The model under review builds one solid part; all positions refer to its coordinate system, in mm. A direction names the side the tool comes from. Round coordinates to 2 decimals unless told otherwise and drop trailing zeros. Write each loop counter-clockwise with the first axis right and the second up, starting at its lowest first coordinate (ties: lowest second). Pieces come first, ordered by that corner, then holes. Notation, with made-up numbers: (34, 41.25) - (63, 41.25) arc R16 ccw to (63, 70.25) - close; hole circle Ø2 at (3.5, -16). An arc over 180 degrees is marked (long way). Use one line per item in the form item = value.
from build123d import *

# Parameters (mm, degrees)
SKETCH_1_R                = 27.5
EXTRUDE_1_DEPTH           = 60
EXTRUDE_1_DEPTH_BACK      = 50
SKETCH_10_W               = 6
SKETCH_10_H               = 40
CUT_EXTRUDE_8_DEPTH       = 8.1
SKETCH_10_2_W             = 6
SKETCH_10_2_H             = 40
CUT_EXTRUDE_9_DEPTH       = 10
CUT_EXTRUDE_9_DEPTH_BACK  = 10
CUT_EXTRUDE_10_DEPTH      = 54
SKETCH_12_R               = 26.5
CUT_EXTRUDE_11_DEPTH      = 58
CUT_EXTRUDE_11_DEPTH_BACK = 54
SKETCH_13_W               = 13
SKETCH_13_H               = 23.5
CUT_EXTRUDE_12_DEPTH      = 54
SKETCH_14_W               = 5
SKETCH_14_H               = 5
EXTRUDE_2_DEPTH           = 1
EXTRUDE_2_DEPTH_BACK      = 4
SKETCH_15_R               = 1.15
CUT_EXTRUDE_13_DEPTH      = 4
CUT_EXTRUDE_13_DEPTH_BACK = 5


with BuildPart() as part:
    # Sketch 1 → Extrude 1 (new body, two sides)
    with BuildSketch(Plane(origin=(0, 0, 0), x_dir=(1, 0, 0), z_dir=(0, 1, 0))) as extrude_1_sk:
        Circle(SKETCH_1_R)
    extrude(amount=EXTRUDE_1_DEPTH)
    extrude(extrude_1_sk.sketch, amount=-EXTRUDE_1_DEPTH_BACK)

    # Sketch 10 → Cut-Extrude 8 (cut)
    with BuildSketch(Plane(origin=(0, 60, 0), x_dir=(1, 0, 0), z_dir=(0, 1, 0))):
        with Locations((-12, 0)):
            Rectangle(SKETCH_10_W, SKETCH_10_H)
        with Locations((12, 0)):
            Rectangle(SKETCH_10_W, SKETCH_10_H)
    extrude(amount=-CUT_EXTRUDE_8_DEPTH, mode=Mode.SUBTRACT)

    # Sketch 10_2 → Cut-Extrude 9 (cut, two sides)
    with BuildSketch(Plane(origin=(0, 60, 0), x_dir=(1, 0, 0), z_dir=(0, 1, 0))) as cut_extrude_9_sk:
        with Locations((-12, 0)):
            Rectangle(SKETCH_10_2_W, SKETCH_10_2_H)
        with Locations((12, 0)):
            Rectangle(SKETCH_10_2_W, SKETCH_10_2_H)
    extrude(amount=CUT_EXTRUDE_9_DEPTH, mode=Mode.SUBTRACT)
    extrude(cut_extrude_9_sk.sketch, amount=-CUT_EXTRUDE_9_DEPTH_BACK, mode=Mode.SUBTRACT)

    # Sketch 11 → Cut-Extrude 10 (cut)
    with BuildSketch(Plane(origin=(0, 0, 0), x_dir=(1, 0, 0), z_dir=(0, 1, 0))):
        with BuildLine():
            Line((23.587956714, 14.137124816), (-24.13203639, 13.186918505))
            ThreePointArc((-24.13203639, 13.186918505), (0.547474823, -27.494549848), (23.587956714, 14.137124816))
        make_face()
    extrude(amount=-CUT_EXTRUDE_10_DEPTH, mode=Mode.SUBTRACT)

    # Sketch 12 → Cut-Extrude 11 (cut, two sides)
    with BuildSketch(Plane(origin=(0, 0, 0), x_dir=(1, 0, 0), z_dir=(0, 1, 0))) as cut_extrude_11_sk:
        Circle(SKETCH_12_R)
    extrude(amount=CUT_EXTRUDE_11_DEPTH, mode=Mode.SUBTRACT)
    extrude(cut_extrude_11_sk.sketch, amount=-CUT_EXTRUDE_11_DEPTH_BACK, mode=Mode.SUBTRACT)

    # Sketch 13 → Cut-Extrude 12 (cut)
    with BuildSketch(Plane.XY):
        with Locations((0, -24.25)):
            Rectangle(SKETCH_13_W, SKETCH_13_H)
    extrude(amount=-CUT_EXTRUDE_12_DEPTH, mode=Mode.SUBTRACT)

    # Sketch 14 → Extrude 2 (add, two sides)
    with BuildSketch(Plane.XY.offset(-28)) as extrude_2_sk:
        with Locations((0, -38.5)):
            Rectangle(SKETCH_14_W, SKETCH_14_H)
        with Locations((0, -10)):
            Rectangle(SKETCH_14_W, SKETCH_14_H)
    extrude(amount=EXTRUDE_2_DEPTH)
    extrude(extrude_2_sk.sketch, amount=-EXTRUDE_2_DEPTH_BACK)

    # Sketch 15 → Cut-Extrude 13 (cut, two sides)
    with BuildSketch(Plane.XY.offset(-28)) as cut_extrude_13_sk:
        with Locations((0, -10)):
            Circle(SKETCH_15_R)
        with Locations((0, -38.5)):
            Circle(SKETCH_15_R)
    extrude(amount=CUT_EXTRUDE_13_DEPTH, mode=Mode.SUBTRACT)
    extrude(cut_extrude_13_sk.sketch, amount=-CUT_EXTRUDE_13_DEPTH_BACK, mode=Mode.SUBTRACT)


solid = part.part
(1) Add section B-B on y = -33.5. Write out the cut boundary in (x, z).
Geometry results:
outline = (-24.13, -13.19) arc R27.5 ccw to (-6.5, -26.72) - (-6.5, -25.69) arc R26.5 cw to (-22.97, -13.21) - close; (6.5, -26.72) arc R27.5 ccw to (23.59, -14.14) - (22.43, -14.11) arc R26.5 cw to (6.5, -25.69) - close
(2) Add section A-A on z = 0. Write out the cut boundary in (x, y).
Geometry results:
outline = (-27.5, 0) - (-26.5, 0) - (-26.5, 58) - (-15, 58) - (-15, 60) - (-27.5, 60) - close; (-9, 58) - (9, 58) - (9, 60) - (-9, 60) - close; (15, 58) - (26.5, 58) - (26.5, 0) - (27.5, 0) - (27.5, 60) - (15, 60) - close
(3) The part is to be moulded in two halves that separate along X. For faces 1 (the flat face through (0, -7.5, -30)), 2 (the cylindrical face through (-0.249, -39.623, -29.198)), 3 (the flat face through (-2.5, -39, -30)), say which applies: +X half, -X half, draft (parallel to the pull), parting line (faces both ways), or undercut.
Geometry results:
face_1 = draft
face_2 = undercut
face_3 = -X half
(4) Machinability: for faces 4 (the flat face through (2.5, -39, -30)), 5 (the flat face through (0, 60, 0)), 6 (the cylindrical face through (-3.45, 16.756, -26.274)), 7 (the flat face through (0, -36, -29)), 8 (the flat face through (-2.5, -10, -30)), which of the approach directions +Z, -Z, +X, -X, +Y, -Y give a long, thin tool a straight path to every point of the face, cutting with its end or side? Answer none if there is none.
Geometry results:
face_4 = -Z, +X, +Y, -Y
face_5 = +Z, -Z, +X, -X, +Y
face_6 = -Y
face_7 = +Z, -Z
face_8 = -Z, -X, +Y, -Y
(5) Add section D-D on x = 13.5. Write out the cut boundary in (y, z).
Geometry results:
outline = (-50, -23.96) - (60, -23.96) - (60, -20) - (58, -20) - (58, -22.8) - (-50, -22.8) - close; (0, 22.8) - (58, 22.8) - (58, 20) - (60, 20) - (60, 23.96) - (0, 23.96) - close
(6) Add section C-C on x = 0. Write out the cut boundary in (y, z), then the cut area to 3 significant figures.
Geometry results:
outline = (-50, -27.5) - (-41, -27.5) - (-41, -32) - (-39.65, -32) - (-39.65, -26.5) - (-50, -26.5) - close; (-37.35, -32) - (-36, -32) - (-36, -26.5) - (-37.35, -26.5) - close; (-12.5, -32) - (-11.15, -32) - (-11.15, -26.5) - (-12.5, -26.5) - close; (-8.85, -32) - (-7.5, -32) - (-7.5, -27.5) - (60, -27.5) - (60, 27.5) - (0, 27.5) - (0, 26.5) - (58, 26.5) - (58, -26.5) - (-8.85, -26.5) - close
area = 272 mm2
(7) Insertion check: P1, Ø5, axis at y = -9.5, z = -30, coming from the -X side; P2, Ø0.6, axis at y = 59, z = 2, coming from the -X side; P3, Ø4, axis at x = 0, y = 47, coming from the -Z side. Each pin has a flat end and moves straight along its axis. Give the tip position at first contact, or say it passes through.
Geometry results:
P1 = -2.5
P2 = -27.45
P3 = -27.5
(8) To check wall thickness, follow L1, parallel to Y at x = 0, z = -28.6; L2, parallel to Y at x = 0, z = -27; L3, parallel to X at y = -38.5, z = -30.35. State the ranges of each line that lie inside material, in increasing order.
Geometry results:
L1 = -41 to -39.65, -37.35 to -36, -12.5 to -11.15, -8.85 to -7.5
L2 = -50 to -39.65, -37.35 to -36, -12.5 to -11.15, -8.85 to 60
L3 = -2.5 to -1.15, 1.15 to 2.5
